from build123d import *

# Parameters (mm, degrees)
F1_DEPTH = 40
F2_R     = 39.99999
F3_R     = 20
F5_D     = 20
F6_R     = 5
F8_DEPTH = 10.001


# Not quite as in the source:
# - a fillet or chamfer is up to 0.001 mm smaller than in the source, because OpenCascade refuses the exact size


with BuildPart() as f1:
    # F0 (on Front) → F1 (new body, symmetric)
    with BuildSketch(Plane.XZ):
        Polygon((0, 10), (0, 0), (150, 0), (190, 69.2820323028), (181.3397459622, 74.2820323028), (151.3397459622, 22.3205080757), (134.0192378865, 32.3205080757), (164.0192378865, 84.2820323028), (155.3589838486, 89.2820323028), (109.5854811567, 10), align=None)
    extrude(amount=F1_DEPTH, both=True)

    # F2 (radius 40 in the source; OpenCascade refuses exactly that, so slightly less here)
    f2_edges = [f1.edges().sort_by_distance(p)[0] for p in [
        (159.689111, -40, 86.782032),
        (159.689111, 40, 86.782032),
        (185.669873, 40, 71.782032),
        (185.669873, -40, 71.782032),
    ]]
    fillet(f2_edges, radius=F2_R)

    # F3
    f3_edges = [f1.edges().sort_by_distance(p)[0] for p in [
        (0, -40, 5),
        (0, 40, 5),
    ]]
    fillet(f3_edges, radius=F3_R)

    # F5 (through all)
    with Locations(Plane(origin=(77.8589838486, 0, -44.9519052838), x_dir=(0, -1, 0), z_dir=(-0.8660254038, 0, 0.5))):
        with Locations((0, 112.1529946162)):
            Hole(F5_D / 2)

    # F6
    f6_edges = [f1.edges().sort_by_distance(p)[0] for p in [
        (109.585481, 0, 10),
    ]]
    fillet(f6_edges, radius=F6_R)

    # F7 (on face) → F8 (cut, through all)
    with BuildSketch(Plane.XY.offset(10)):
        with BuildLine():
            Line((0, 0), (0, -10))
            Line((0, -10), (60, -10))
            ThreePointArc((60, -10), (70, 0), (60, 10))
            Line((60, 10), (0, 10))
            Line((0, 10), (0, 0))
        make_face()
    extrude(amount=-F8_DEPTH, mode=Mode.SUBTRACT)


solid = f1.part
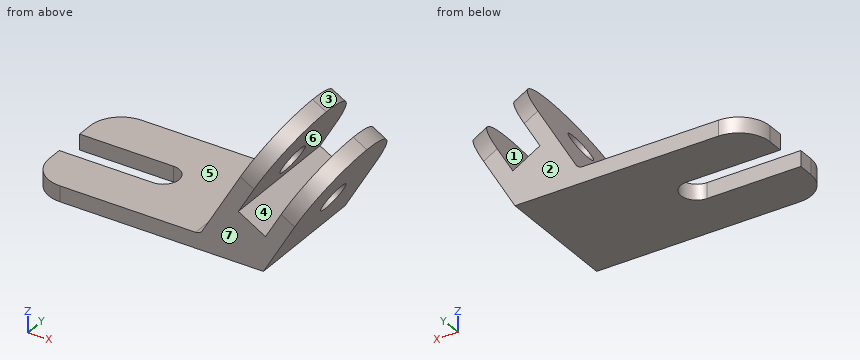
The model under review builds one solid part; all positions refer to its coordinate system, in mm. Face numbers are marked on the shaded views. A direction names the side the tool comes from. Coordinates: 2 decimals unless noted, no trailing zeros. Write each loop counter-clockwise with the first axis right and the second up, starting at its lowest first coordinate (ties: lowest second). Pieces come first, ordered by that corner, then holes. Notation, with made-up numbers: M 41,-11 L 53,-11 A6 cw 53,0 Z; hole C 53,73.5 d11. An arc over 180 degrees is marked long. Put each result on its own line as item: value.
1) Clearance check with flat-ended pins moving along their axes: pin 1 Ø1 at (y, z) = (0, 19.5) entering from +X; pin 2 Ø10 at (y, z) = (-7, 28) entering from -X; pin 3 Ø3 at (y, z) = (-15.5, 64) entering from +X. State where each tip first meets the part, or that it passes through.
Computed:
pin 1: stops at x = 161.55
pin 2: stops at x = 117.09
pin 3: stops at x = 187.82
2) Draft analysis for pull direction X (two halves, no side actions). For the marked faces 1, 2, 3 and 4, state which applies: released by +X, released by -X, zero draft, split by the parting line, or undercut.
Computed:
face 1: undercut
face 2: zero draft
face 3: released by +X
face 4: undercut
3) Add section B-B on y = 6. Give the boundary of the cut face in (x, z).
Computed:
outline: M 68,0 L 150,0 L 164.58,25.25 L 155.92,30.25 L 151.34,22.32 L 134.02,32.32 L 138.6,40.25 L 129.94,45.25 L 111.03,12.5 A5 cw 106.7,10 L 68,10 Z; M 137.94,59.1 L 146.6,54.1 L 163.79,83.89 L 155.13,88.89 Z; M 163.92,44.1 L 172.58,39.1 L 189.77,68.89 L 181.11,73.89 Z
4) Wall thickness on probe 1 along Z at (x, y) = (99, -1); probe 2 along Z at (x, y) = (144.5, 30); probe 3 along X at (y, z) = (-24.5, 46): over which ranges is each line inside the solid? List them lowest first. Write a range as [from, to].
Computed:
probe 1: z = [0, 10]
probe 2: z = [0, 26.27], [50.47, 70.47]
probe 3: x = [130.37, 141.92], [165.01, 176.56]
5) Add section D-D on x = 82.5. Give the boundary of the cut face in (y, z), then the cut area to 3 significant figures.
Computed:
outline: M -40,0 L 40,0 L 40,10 L -40,10 Z
area: 800 mm2
6) For the marked faces 5, 6 and 7, list the 3-axis set-ups (+Z, -Z, +X, -X, +Y, -Y) from which the entire face can be reached by the end or side of a thin tool; tool diameter is ignored.
Computed:
face 5: +Z, -X, +Y, -Y
face 6: +Y, -Y
face 7: +Z, -Z, +X, -X, -Y
7) Add section A-A on x = 36.5. Give the boundary of the cut face in (y, z), then the cut area to 3 significant figures.
Computed:
outline: M -40,0 L -10,0 L -10,10 L -40,10 Z; M 10,0 L 40,0 L 40,10 L 10,10 Z
area: 600 mm2
8) Add section C-C on y = -17. Give the boundary of the cut face in (x, z).
Computed:
outline: M 0,0 L 150,0 L 188.1,66 L 179.44,71 L 151.34,22.32 L 134.02,32.32 L 162.12,81 L 153.46,86 L 111.03,12.5 A5 cw 106.7,10 L 0,10 Z
